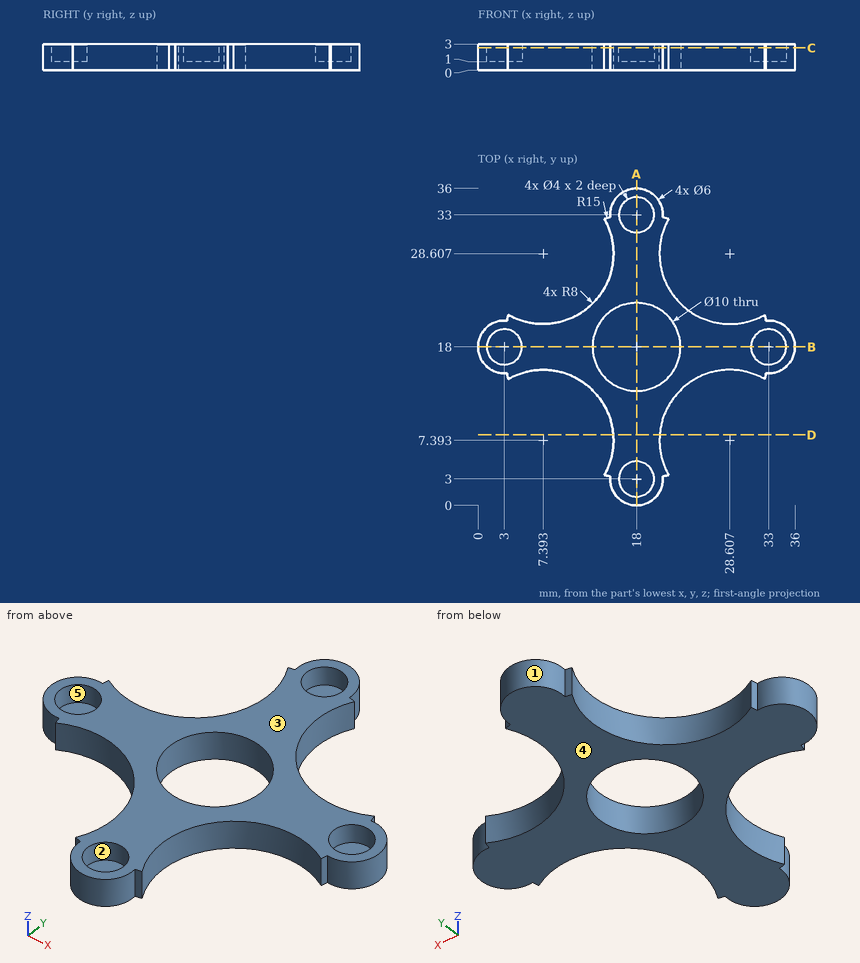
Can you work these out from the drawing? Everything is in mm from the part's minimum corner. A direction names the side the tool comes from. Give positions to 0.01 mm unless a question says otherwise; leave off trailing zeros. Order: outer loops, then holes, each group sorted by start corner. A loop starts at its lowest first (then second) coordinate and runs counter-clockwise, first axis right, second up.
1. Suppose I cut it at D-D (y = 8). List the corners of the cut face in (x, z) for me.
2. We'd pull the mould along X, two halves only. Please class the marked faces 1, 2 and 3: pulls with the +X half, pulls with the -X half, needs draft (parallel to the pull), parting line crosses it, or undercut.
3. Suppose I cut it at A-A (x = 18). List the corners of the cut face in (y, z) for me.
4. I need wall thicknesses on L1, parallel to Y at x = 18, z = 1.8; L2, parallel to Y at x = 33, z = 2.2; L3, parallel to Y at x = 13.5, z = 0.55 (1 decimal). Which ranges of each line are inside material? Lowest first, please.
5. For the marked faces 4 and 5, which set-ups out of +Z, -Z, +X, -X, +Y, -Y let a thin tool reach every point of the face, with its end or its side?
6. Suppose I cut it at C-C (z = 2.55). Give the number of separate pieces and of enclosed holes in the cut face, plus the area to 3 significant figures.
7. Will these pins go through, and if not, where does the flat tip stop? P1, Ø1.2, axis at x = 32, y = 18.5, coming from the +Z side; P2, Ø1.5, axis at x = 25.5, z = 1.5, coming from the -Y side; P3, Ø1, axis at y = 21, z = 0.5, coming from the -X side.
Solved:
1. outline: (15.37, 0) - (20.63, 0) - (20.63, 3) - (15.37, 3) - close
2. face 1: parting line crosses it
2. face 2: undercut
2. face 3: needs draft
3. outline: (0, 0) - (13, 0) - (13, 3) - (5, 3) - (5, 1) - (1, 1) - (1, 3) - (0, 3) - close; (23, 0) - (36, 0) - (36, 3) - (35, 3) - (35, 1) - (31, 1) - (31, 3) - (23, 3) - close
4. L1: y = 0 to 1, 5 to 13, 23 to 31, 35 to 36
4. L2: y = 15 to 16, 20 to 21
4. L3: y = 12.6 to 15.8, 20.2 to 23.4
5. face 4: -Z, +X, -X, +Y, -Y
5. face 5: +Z
6. separate pieces: 1
6. enclosed holes: 5
6. area: 281 mm2
7. P1: stops at z = 1
7. P2: stops at y = 14.4
7. P3: stops at x = 1.34
